```python
from build123d import *

# Parameters (mm, degrees)
SKETCH1_R           = 1.5
BOSS_EXTRUDE1_DEPTH = 1.6


with BuildPart() as part:
    # Sketch1 → Boss-Extrude1 (new body)
    with BuildSketch(Plane(origin=(0, 0, 0), x_dir=(1, 0, 0), z_dir=(0, 1, 0))):
        with BuildLine():
            Line((-9.702113495, 11.642067097), (-9.702113495, 12.55))
            ThreePointArc((-9.702113495, 12.55), (-9.497088242, 13.044974747), (-9.002113495, 13.25))
            Line((-9.002113495, 13.25), (13.797886505, 13.25))
            ThreePointArc((13.797886505, 13.25), (15.212100067, 12.664213562), (15.797886505, 11.25))
            Line((15.797886505, 11.25), (15.797886505, -11.25))
            ThreePointArc((15.797886505, -11.25), (15.212100067, -12.664213562), (13.797886505, -13.25))
            Line((13.797886505, -13.25), (-8.850291446, -13.25))
            ThreePointArc((-8.850291446, -13.25), (-9.345266193, -13.044974747), (-9.550291446, -12.55))
            Line((-9.550291446, -12.55), (-9.550291446, -11.824237104))
            ThreePointArc((-9.550291446, -11.824237104), (-9.7553167, -11.329262357), (-10.250291446, -11.124237104))
            Line((-10.250291446, -11.124237104), (-16.202113495, -11.124237104))
            Line((-16.202113495, -11.124237104), (-16.202113495, -5.604412091))
            Line((-16.202113495, -5.604412091), (-16.152113495, -5.604412091))
            ThreePointArc((-16.152113495, -5.604412091), (-15.657138749, -5.399386838), (-15.452113495, -4.904412091))
            Line((-15.452113495, -4.904412091), (-15.452113495, 3.695587909))
            ThreePointArc((-15.452113495, 3.695587909), (-15.657138749, 4.190562656), (-16.152113495, 4.395587909))
            Line((-16.152113495, 4.395587909), (-16.202113495, 4.395587909))
            Line((-16.202113495, 4.395587909), (-16.202113495, 10.942067097))
            Line((-16.202113495, 10.942067097), (-10.402113495, 10.942067097))
            ThreePointArc((-10.402113495, 10.942067097), (-9.907138749, 11.14709235), (-9.702113495, 11.642067097))
        make_face()
        with Locations((12.797886505, 10.5)):
            Circle(SKETCH1_R, mode=Mode.SUBTRACT)
        with Locations((12.797886505, -10.5)):
            Circle(SKETCH1_R, mode=Mode.SUBTRACT)
    extrude(amount=BOSS_EXTRUDE1_DEPTH)


solid = part.part
```
Read the model definition and answer for the solid it produces. Units are mm, in the model's axes. A direction names the side the tool comes from. Coordinates: 2 decimals unless noted, no trailing zeros. Loops run counter-clockwise (first coordinate to the right, second up) from the corner with the lowest first, then second, coordinate; pieces in that order, holes last.
(1) Flat-ended cylindrical pins translate along their axes: pin 1 Ø0.5 at (x, y) = (-12, 1) entering from -Z; pin 2 Ø0.5 at (y, z) = (1, -12) entering from -X. Find the tip coordinate at first contact, or state that the pin passes through.
Solution:
pin 1: stops at z = -10.94
pin 2: stops at x = -9.7
(2) The part is cut by section A-A (z = -10.5). Determine the outline of the cut face in (x, y), and give its area (3 significant figures).
Solution:
outline: (-16.2, 0) - (11.3, 0) - (11.3, 1.6) - (-16.2, 1.6) - close; (14.3, 0) - (15.8, 0) - (15.8, 1.6) - (14.3, 1.6) - close
area: 46.4 mm2
(3) The part is cut by section B-B (y = 0.5). Determine the outline of the cut face in (x, z), and give its area (3 significant figures).
Solution:
outline: (-16.2, -10.94) - (-10.4, -10.94) arc R0.7 cw to (-9.7, -11.64) - (-9.7, -12.55) arc R0.7 ccw to (-9, -13.25) - (13.8, -13.25) arc R2 ccw to (15.8, -11.25) - (15.8, 11.25) arc R2 ccw to (13.8, 13.25) - (-8.85, 13.25) arc R0.7 ccw to (-9.55, 12.55) - (-9.55, 11.82) arc R0.7 cw to (-10.25, 11.12) - (-16.2, 11.12) - (-16.2, 5.6) - (-16.15, 5.6) arc R0.7 cw to (-15.45, 4.9) - (-15.45, -3.7) arc R0.7 cw to (-16.15, -4.4) - (-16.2, -4.4) - close; hole circle Ø3 at (12.8, -10.5); hole circle Ø3 at (12.8, 10.5)
area: 796 mm2
(4) The mould has two halves that part along Z. Classify faces 1 (the face through (15.196, 0.789, -12.68)), 2 (the face through (-9.702, 1, -12)), 3 (the face through (14.184, 0.789, 11.075)), 4 (the face through (15.228, 0.789, 12.649)): released by +Z, released by -Z, zero draft, split by the parting line, or undercut.
Solution:
face 1: released by -Z
face 2: zero draft
face 3: undercut
face 4: released by +Z
(5) The part is cut by section C-C (x = 12.5). Determine the outline of the cut face in (y, z).
Solution:
outline: (0, -13.25) - (1.6, -13.25) - (1.6, -11.97) - (0, -11.97) - close; (0, -9.03) - (1.6, -9.03) - (1.6, 9.03) - (0, 9.03) - close; (0, 11.97) - (1.6, 11.97) - (1.6, 13.25) - (0, 13.25) - close
(6) A tool of negligible diameter and unlimited length cuts with its end or side. For faces 5 (the face through (-15.452, 1, 1)), 6 (the face through (-13, 1, 11.124)), 7 (the face through (-13, 1, -10.942)), from which of +Z, -Z, +X, -X, +Y, -Y can it reach the whole face along a straight path? Write none if from no direction.
Solution:
face 5: -X, +Y, -Y
face 6: +Z, -X, +Y, -Y
face 7: -Z, -X, +Y, -Y
(7) Consider line 1 along X through (y, z) = (0.65, -10.5); line 2 along Z through (x, y) = (-12, 1.3); line 3 along X through (y, z) = (1, -10). Determine where each line is inside the solid, lowest interval first.
Solution:
line 1: x = -16.2 to 11.3, 14.3 to 15.8
line 2: z = -10.94 to 11.12
line 3: x = -16.2 to 11.38, 14.21 to 15.8
